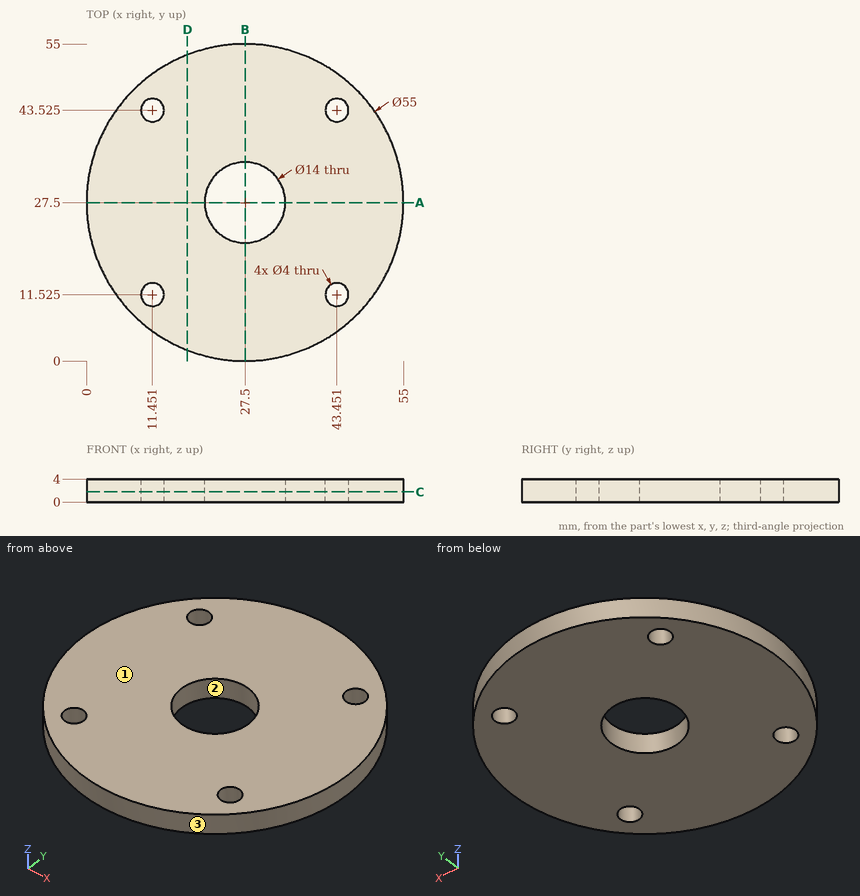
Study the drawing (mm; zero at the part's minimum x, y, z) and answer. Coordinates: 2 decimals unless noted, no trailing zeros. Loops run counter-clockwise (first coordinate to the right, second up) from the corner with the lowest first, then second, coordinate; pieces in that order, holes last. Notation, with made-up numbers: M -26.75,-16 L -13.75,-16 A18 cw -13.75,2 Z; hole C -15,36.5 d7. An arc over 180 degrees is marked long. Answer in a Markdown table with one row per item.
1) Find section A-A (y = 27.5). Determine the outline of the cut face in (x, z), then the cut area to 3 significant figures.
Answers below:
| item | result |
|---|---|
| outline | M 0,0 L 20.5,0 L 20.5,4 L 0,4 Z; M 34.5,0 L 55,0 L 55,4 L 34.5,4 Z |
| area | 164 mm^2 |
2) Given pin 1 (1.5 mm diameter, centred on y = 35.5, z = 1.5, fed in from +X); pin 2 (2 mm diameter, centred on y = 18, z = 2.5, fed in from -X); pin 3 (2 mm diameter, centred on x = 12.5, z = 2.5, fed in from -Y), each flat-ended and moving along its own axis, determine where each tip first touches the part or whether it passes through.
Answers below:
| item | result |
|---|---|
| pin 1 | x = 54.03 |
| pin 2 | x = 1.35 |
| pin 3 | y = 3.83 |
3) Find section D-D (x = 17.5). Determine the outline of the cut face in (y, z), then the cut area to 3 significant figures.
Answers below:
| item | result |
|---|---|
| outline | M 1.88,0 L 53.12,0 L 53.12,4 L 1.88,4 Z |
| area | 205 mm^2 |
4) Determine the mould class of the marked faces 1, 2 and 3 for opening direction Y: released by +Y, released by -Y, zero draft, split by the parting line, or undercut.
Answers below:
| item | result |
|---|---|
| face 1 | zero draft |
| face 2 | undercut |
| face 3 | split by the parting line |
5) Find the intervals of material crossed by probe 1 along X at (y, z) = (13, 3.85) (1 decimal); probe 2 along Y at (x, z) = (27.5, 1.4); probe 3 along X at (y, z) = (10.5, 3.4) (1 decimal), in increasing order.
Answers below:
| item | result |
|---|---|
| probe 1 | 4.1 to 10.1, 12.8 to 42.1, 44.8 to 50.9 |
| probe 2 | 0 to 20.5, 34.5 to 55 |
| probe 3 | 5.9 to 9.7, 13.2 to 41.7, 45.2 to 49.1 |
6) Find section C-C (z = 1.75). Count the separate pieces of the cut face and the enclosed holes in it, then the cut area to 3 significant figures.
Answers below:
| item | result |
|---|---|
| separate pieces | 1 |
| enclosed holes | 5 |
| area | 2,170 mm^2 |
